Read the model definition and answer for the solid it produces. Units are mm, in the model's axes. Give positions to 0.01 mm unless a question says otherwise; leave off trailing zeros. Write each loop counter-clockwise with the first axis right and the second up, starting at its lowest first coordinate (ties: lowest second). Pieces come first, ordered by that corner, then holes. Notation, with made-up numbers: M 62,-34 L 90,-34 A19 cw 90,-26 Z; hole C 62.5,72.25 d1. An arc over 180 degrees is marked long. Use a Markdown table: item, result. Add a question column.
Item 1: Consider probe 1 along X at (y, z) = (16, 12); probe 2 along Z at (x, y) = (88.9, 18) (3 decimals); probe 3 along Z at (x, y) = (529.5, 244.5). Determine where each line is inside the solid, lowest interval first. Write a range as [from, to].
Item 2: A cutting plane is placed at B-B on y = 266.5. Determine the outline of the cut face in (x, z), then the cut area to 3 significant figures.
Item 3: Given P1, Ø12.5, axis at y = 6.5, z = 16.5, coming from the +X side; P2, Ø8, axis at x = 222.5, y = 304.5, coming from the -Z side; P3, Ø8, axis at y = 158.5, z = 19.5, coming from the +X side, each flat-ended and moving along its own axis, determine where each tip first touches the part or whether it passes through.
Item 4: A cutting plane is placed at A-A on x = 466.5. Determine the outline of the cut face in (y, z), then the cut area to 3 significant figures.
from build123d import *

# Parameters (mm, degrees)
F1_DEPTH = 457.2
F0_W     = 25.4
F0_H     = 25.4
F0_R     = 3.175
F2_DEPTH = 25.4
F3_START = -431.8
F3_DEPTH = 25.4
F4_START = -12.7
F4_DEPTH = 431.8


with BuildPart() as f1:
    # F0 (on Front) → F1 (new body)
    with BuildSketch(Plane.XZ):
        Polygon((711.2, 63.5), (0, 63.5), (0, 25.4), (76.2, 25.4), (101.6, 25.4), (609.6, 25.4), (635, 25.4), (711.2, 25.4), align=None)
    extrude(amount=-F1_DEPTH)

    # F0 (on Front) → F2 (join)
    with BuildSketch(Plane.XZ):
        with Locations((88.9, 12.7)):
            Rectangle(F0_W, F0_H)
        with Locations((88.9, 12.7)):
            Circle(F0_R, mode=Mode.SUBTRACT)
        with Locations((622.3, 12.7)):
            Rectangle(F0_W, F0_H)
        with Locations((622.3, 12.7)):
            Circle(F0_R, mode=Mode.SUBTRACT)
        with Locations((88.9, 12.7)):
            Circle(F0_R)
        with Locations((622.3, 12.7)):
            Circle(F0_R)
    extrude(amount=-F2_DEPTH)

    # F0 (on Front) → F3 (join)
    with BuildSketch(Plane.XZ.offset(F3_START)):
        with Locations((88.9, 12.7)):
            Rectangle(F0_W, F0_H)
        with Locations((88.9, 12.7)):
            Circle(F0_R, mode=Mode.SUBTRACT)
        with Locations((622.3, 12.7)):
            Rectangle(F0_W, F0_H)
        with Locations((622.3, 12.7)):
            Circle(F0_R, mode=Mode.SUBTRACT)
        with Locations((622.3, 12.7)):
            Circle(F0_R)
        with Locations((88.9, 12.7)):
            Circle(F0_R)
    extrude(amount=-F3_DEPTH)

    # F0 (on Front) → F4 (cut)
    with BuildSketch(Plane.XZ.offset(F4_START)):
        with Locations((88.9, 12.7)):
            Circle(F0_R)
        with Locations((622.3, 12.7)):
            Circle(F0_R)
    extrude(amount=-F4_DEPTH, mode=Mode.SUBTRACT)


solid = f1.part
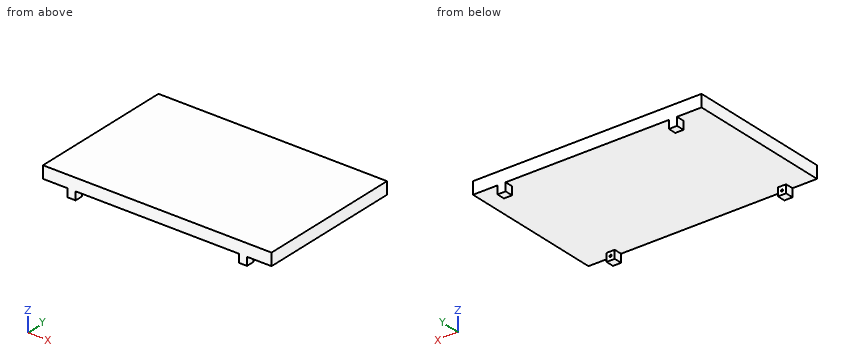
Filled in:
| question | item | result |
|---|---|---|
| 1 | probe 1 | [76.2, 85.8], [92, 101.6], [609.6, 619.2], [625.4, 635] |
| 1 | probe 2 | [0, 9.525], [15.875, 63.5] |
| 1 | probe 3 | [25.4, 63.5] |
| 2 | outline | M 0,25.4 L 711.2,25.4 L 711.2,63.5 L 0,63.5 Z |
| 2 | area | 27,100 mm² |
| 3 | P1 | x = 635 |
| 3 | P2 | z = 25.4 |
| 3 | P3 | through |
| 4 | outline | M 0,25.4 L 457.2,25.4 L 457.2,63.5 L 0,63.5 Z |
| 4 | area | 17,400 mm² |
